Input: part model. Units: mm. Frame: model coordinates. Face numbers are marked on the shaded views. A direction names the side the tool comes from. Coordinates: 2 decimals unless noted, no trailing zeros. Order: outer loops, then holes, each group sorted by start corner. A loop starts at its lowest first (then second) coordinate and runs counter-clockwise, first axis right, second up. Notation, with made-up numbers: M 24,-32.75 L 57,-32.75 A10 cw 57,-22.75 Z; hole C 48,-0.75 d10. An arc over 180 degrees is marked long. One line per item, written item: value.
```python
from build123d import *

# Parameters (mm, degrees)
SKETCH1_R          = 3.175
EXTRUDE1_DEPTH     = 12.7
CHAMFER3_SIZE      = 0.9525
SKETCH6_R          = 4.7625
EXTRUDE2_DEPTH     = 6.35
CUT_EXTRUDE1_DEPTH = 3.571875
CHAMFER1_SIZE      = 0.47625
CHAMFER2_SIZE      = 0.238125


with BuildPart() as part:
    # Sketch1 → Extrude1 (new body)
    with BuildSketch(Plane.XY):
        Circle(SKETCH1_R)
    extrude(amount=-EXTRUDE1_DEPTH)

    # Chamfer3
    chamfer3_edges = [part.edges().sort_by_distance(p)[0] for p in [
        (-3.175, 0, 0),
    ]]
    chamfer(chamfer3_edges, length=CHAMFER3_SIZE)

    # Sketch6 → Extrude2 (add)
    with BuildSketch(Plane(origin=(0, 0, -12.7), x_dir=(-1, 0, 0), z_dir=(0, 0, -1))):
        Circle(SKETCH6_R)
    extrude(amount=EXTRUDE2_DEPTH)

    # Sketch7 → Cut-Extrude1 (cut)
    with BuildSketch(Plane(origin=(0, 0, -19.05), x_dir=(-1, 0, 0), z_dir=(0, 0, -1))):
        Polygon((0, 2.749630657), (-2.38125, 1.374815329), (-2.38125, -1.374815329), (0, -2.749630657), (2.38125, -1.374815329), (2.38125, 1.374815329), align=None)
    extrude(amount=-CUT_EXTRUDE1_DEPTH, mode=Mode.SUBTRACT)

    # Chamfer1
    chamfer1_edges = [part.edges().sort_by_distance(p)[0] for p in [
        (4.7625, 0, -19.05),
    ]]
    chamfer(chamfer1_edges, length=CHAMFER1_SIZE)

    # Chamfer2
    chamfer2_edges = [part.edges().sort_by_distance(p)[0] for p in [
        (4.7625, 0, -12.7),
    ]]
    chamfer(chamfer2_edges, length=CHAMFER2_SIZE)


solid = part.part
```
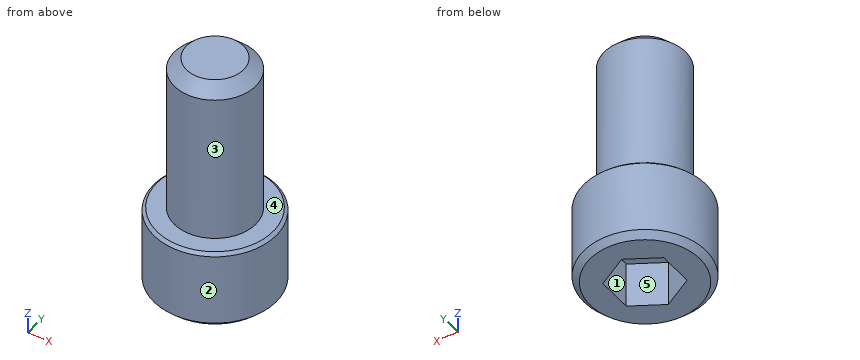
(1) Ray query, line 1 (Z direction, x = 3.75, y = 1.25); line 2 (Z direction, x = 1.25, y = 1.5); line 3 (X direction, y = -1.75, z = -16.25). Return the intervals inside material, ascending. Write a range as from..to.
Data:
line 1: z = -19.05..-12.7
line 2: z = -15.48..0
line 3: x = -4.43..-1.73, 1.73..4.43
(2) Access query for the marked faces 1 and 2. Directions: +Z, -Z, +X, -X, +Y, -Y. A direction counts if a zero-diameter tool reaches every point of the face in a straight line with its end or side. Return the directions, or none.
Data:
face 1: -Z
face 2: +Z, -Z
(3) Cut plane B-B on z = -4. Output: boundary loops of the cut face in (x, y) (3 decimals).
Data:
outline: C 0,0 d6.35
(4) Draft query along X for the marked faces 3, 4 and 5. Return one class per face: released by +X, released by -X, zero draft, split by the parting line, or undercut.
Data:
face 3: split by the parting line
face 4: zero draft
face 5: undercut
(5) First-contact query: pin 1 (2 mm diameter, centred on y = 1.5, z = -4, fed in from +X); pin 2 (1 mm diameter, centred on y = 1, z = -11.5, fed in from -X); pin 3 (2 mm diameter, centred on x = 3, z = -11.5, fed in from -Y). Flat tips, straight axial feed; report the tip coordinate or a pass-through.
Data:
pin 1: stops at x = 3.14
pin 2: stops at x = -3.14
pin 3: stops at y = -2.47
